```python
from build123d import *

# Parameters (mm, degrees)
SKETCH1_R           = 4
BOSS_EXTRUDE1_DEPTH = 10
SKETCH2_R           = 4
BOSS_EXTRUDE2_DEPTH = 10


with BuildPart() as part:
    # Sketch1 → Boss-Extrude1 (new body)
    with BuildSketch(Plane(origin=(0, 0, 0), x_dir=(0, 0, -1), z_dir=(1, 0, 0))):
        with BuildLine():
            Line((10, 70), (10, 10))
            Line((10, 10), (0, 10))
            ThreePointArc((0, 10), (-10, 0), (0, -10))
            Line((0, -10), (10, -10))
            Line((10, -10), (10, -70))
            Line((10, -70), (15, -70))
            Line((15, -70), (15, 70))
            Line((15, 70), (10, 70))
        make_face()
        Circle(SKETCH1_R, mode=Mode.SUBTRACT)
    extrude(amount=BOSS_EXTRUDE1_DEPTH)

    # Sketch2 → Boss-Extrude2 (add)
    with BuildSketch(Plane(origin=(0, 0, -15), x_dir=(-1, 0, 0), z_dir=(0, 0, -1))):
        with Locations((-5, 65)):
            Circle(SKETCH2_R)
        with Locations(Location((-5, -65, 0), (0, 0, 180))):
            Circle(SKETCH2_R)
    extrude(amount=BOSS_EXTRUDE2_DEPTH)


solid = part.part
```
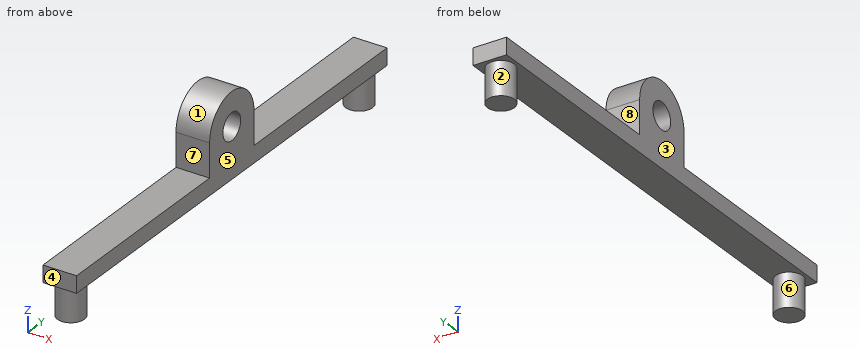
Could you check a few things on this model? Use its own coordinates, in mm. Face numbers are marked on the shaded views. A direction names the side the tool comes from. Coordinates: 2 decimals unless noted, no trailing zeros. Write each loop counter-clockwise with the first axis right and the second up, starting at its lowest first coordinate (ties: lowest second). Pieces come first, ordered by that corner, then holes. Notation, with made-up numbers: (26.5, 32.5) -> (45.5, 32.5) arc R17 cw to (45.5, 49.5) -> close; hole circle Ø9 at (75, 62). An arc over 180 degrees is marked (long way). Return JSON: item names as keys, results as strings.
(1) Imagine slicing it at A-A, the plane y = 0. Please give me the cut outline in (x, z), then the cut area to 3 significant figures.
Numbers:
{"outline": "(0, -15) -> (10, -15) -> (10, -4) -> (0, -4) -> close; (0, 4) -> (10, 4) -> (10, 10) -> (0, 10) -> close", "area": "170 mm2"}
(2) Imagine slicing it at B-B, the plane x = 5. Please give me the cut outline in (y, z), then the cut area to 3 significant figures.
Numbers:
{"outline": "(-70, -15) -> (-69, -15) -> (-69, -25) -> (-61, -25) -> (-61, -15) -> (61, -15) -> (61, -25) -> (69, -25) -> (69, -15) -> (70, -15) -> (70, -10) -> (10, -10) -> (10, 0) arc R10 ccw to (-10, 0) -> (-10, -10) -> (-70, -10) -> close; hole circle Ø8 at (0, 0)", "area": "1,170 mm2"}
(3) We'd pull the mould along Y, two halves only. Please class the marked faces 1, 2 and 3: +Y half, -Y half, draft (parallel to the pull), parting line (faces both ways), or undercut.
Numbers:
{"face 1": "parting line", "face 2": "undercut", "face 3": "draft"}
(4) I need wall thicknesses on L1, parallel to Y at x = 4, z = -6; L2, parallel to Z at x = 9, y = 62; L3, parallel to Y at x = 5.5, z = 3. Which ranges of each line are inside material? Lowest first, please.
Numbers:
{"L1": "y = -10 to 10", "L2": "z = -15 to -10", "L3": "y = -9.54 to -2.65, 2.65 to 9.54"}
(5) Imagine slicing it at D-D, the plane z = -7.5. Please give me the cut outline in (x, y), then the cut area to 3 significant figures.
Numbers:
{"outline": "(0, -10) -> (10, -10) -> (10, 10) -> (0, 10) -> close", "area": "200 mm2"}
(6) Which directions (+Z, -Z, +X, -X, +Y, -Y) give clear straight access to the entire face, cutting with the end or side of a thin tool? Please do the marked faces 4, 5, 6, 7 and 8.
Numbers:
{"face 4": "+Z, -Z, +X, -X, -Y", "face 5": "+Z, -Z, +X, +Y, -Y", "face 6": "-Z", "face 7": "+Z, +X, -X, -Y", "face 8": "+Z, +X, -X, +Y"}
(7) Imagine slicing it at C-C, the plane y = 65. Please give me the cut outline in (x, z).
Numbers:
{"outline": "(0, -15) -> (1, -15) -> (1, -25) -> (9, -25) -> (9, -15) -> (10, -15) -> (10, -10) -> (0, -10) -> close"}
(8) I'm going to push flat-ended pins straight in: pin 1 (1 mm diameter, centred on x = 7.5, z = -3, fed in from +Y); pin 2 (3 mm diameter, centred on x = 7, z = -7, fed in from -Y); pin 3 (1 mm diameter, centred on x = 7.5, y = -42, fed in from +Z). Where does each tip first touch, or does it pass through?
Numbers:
{"pin 1": "stops at y = 10", "pin 2": "stops at y = -10", "pin 3": "stops at z = -10"}
